Autodesk Inventor part; units mm, degrees
ref_plane "YZ Plane" through (0, 0, 0) normal (1, 0, 0) x (0, 1, 0)
ref_plane "XZ Plane" through (0, 0, 0) normal (0, 1, 0) x (-1, 0, 0)
ref_plane "XY Plane" through (0, 0, 0) normal (0, 0, 1) x (1, 0, 0)
sketch "Sketch1" plane through (0, 0, 0) normal (0, 0, 1) x (1, 0, 0)
  line L0 (0.0426, 8.3509) -> (2.1366, 8.3509) construction
  line L1 (-5.93, 6.5274) -> (-3.3043, 9.5646)
  line L2 (-3.3043, 9.5646) -> (-1.75, 9.5646)
  line L3 (-1.75, 9.5646) -> (-1.75, 6.9793)
  line L4 (-1.75, 6.9793) -> (0, 8.1293)
  line L5 (0, 8.1293) -> (0, 0)
  line L6 (0, 0) -> (-1.75, 1.15)
  line L7 (-1.75, 1.15) -> (-1.75, -1.4354)
  line L8 (-1.75, -1.4354) -> (-3.3043, -1.4354)
  line L9 (-3.3043, -1.4354) -> (-5.93, 1.6019)
  line L10 (-5.93, 1.6019) -> (-5.93, 6.5274)
  dimension "d16" = 0
  dimension "d17" = 0
extrude "Extrusion1" add sketch "Sketch1" along normal blind 164.9
sketch "Sketch2" plane through (0, 0, 0) normal (1, 0, 0) x (0, 0, -1)
  line L0 (0, 8.1293) -> (-164.9, 8.1293)
  line L1 (0, 0) -> (0, 8.1293)
  line L2 (-164.9, 8.1293) -> (0, 8.1293)
  line L3 (0, 8.1293) -> (0, 0)
  line L4 (0, 0) -> (-164.9, 0)
  line L5 (-164.9, 0) -> (-164.9, 8.1293)
extrude "Extrusion2" add sketch "Sketch2" along normal blind 1
sketch "Sketch3" plane through (1, 0, 0) normal (1, 0, 0) x (0, 0, -1)
  line L0 (-164.9, 8.1293) -> (-164.9, 0)
  line L1 (0, 2.065) -> (-164.9, 2.065)
  line L2 (-164.9, 2.065) -> (-164.9, 6.065)
  line L3 (-164.9, 6.065) -> (0, 6.065)
  line L4 (0, 6.065) -> (0, 2.065)
  line L5 (0, 2.065) -> (-164.9, 6.065) construction
  line L6 (-164.9, 2.065) -> (0, 6.065) construction
  line L7 (0, 0) -> (0, 8.1293)
  point P0 (-82.45, 4.065)
  dimension "d22" = 4
  dimension "d28" = 0
extrude "Extrusion3" add sketch "Sketch3" along normal blind 10.5
sketch "Sketch4" plane through (1, 2.065, 0) normal (0, -1, 0) x (1, 0, 0)
  point P0 (-1, 0)
sketch "Sketch5" plane through (1, 2.065, 0) normal (0, -1, 0) x (1, 0, 0)
  line L0 (0, 164.9) -> (10.5, 164.9)
  line L1 (9.5, -0.1) -> (1, -0.1)
  line L2 (1, -0.1) -> (1, 164.9)
  line L3 (1, 164.9) -> (9.5, 164.9)
  line L4 (9.5, 164.9) -> (9.5, -0.1)
  line L5 (9.5, -0.1) -> (1, 164.9) construction
  line L6 (1, -0.1) -> (9.5, 164.9) construction
  point P0 (-1, 0)
  point P1 (5.25, 82.4)
  dimension "d25" = 8.5
extrude "Extrusion4" cut sketch "Sketch5" against normal blind 0.9
fillet "Fillet1" radius 2 1 edges at (11.5, 6.065, 82.45)
fillet "Fillet2" radius 0.2 1 edges at (10.5, 2.965, 82.45)
fillet "Fillet3" radius 0.2 1 edges at (2, 2.965, 82.45)
fillet "Fillet4" radius 0.2 3 edges at (11.5, 2.065, 82.45) (10.5, 2.065, 82.45) (2, 2.065, 82.45)
properties part number "LED Strip Top Mount"
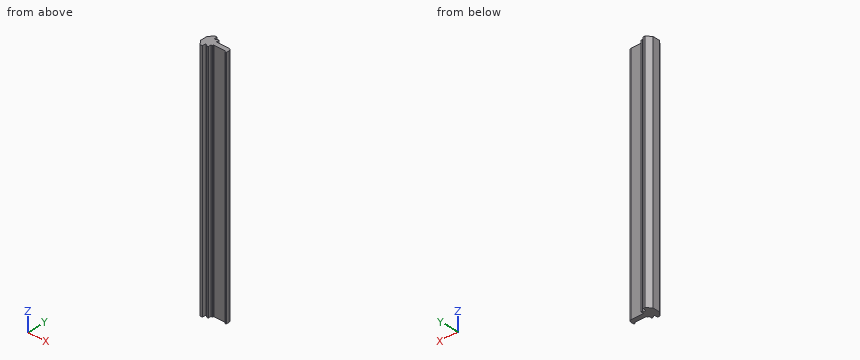
CAD build for the part. Positions are in the model's coordinates, mm. Round coordinates to 2 decimals unless told otherwise and drop trailing zeros. Loops run counter-clockwise (first coordinate to the right, second up) from the corner with the lowest first, then second, coordinate; pieces in that order, holes last.
(1) Drop flat-ended pins along their axis: pin 1 (2 mm diameter, centred on y = 8.5, z = 70.5, fed in from +X); pin 2 (3 mm diameter, centred on x = 0, z = 38.5, fed in from +Y); pin 3 (7 mm diameter, centred on x = 7, z = 47.5, fed in from +Y) (3 decimals). Give the stop position or say it passes through.
(2) Cut at A-A (z = 52). Give the cut face in (x, y) (3 decimals).
(3) Wall check: line 1 along X through (y, z) = (7.5, 21); line 2 along X through (y, z) = (0.5, 119); line 3 along X through (y, z) = (2, 68). Give the ranges that are in metal, low to high.
(4) Cut at B-B (x = 7.75). Give the cut face in (y, z) (3 decimals).
Findings below:
1. pin 1: stops at x = 1
1. pin 2: stops at y = 8.13
1. pin 3: stops at y = 6.065
2. outline: (-5.93, 1.602) - (-3.304, -1.435) - (-1.75, -1.435) - (-1.75, 1.15) - (0, 0) - (1, 0) - (1, 2.065) - (1.8, 2.065) arc R0.2 ccw to (2, 2.265) - (2, 2.765) arc R0.2 cw to (2.2, 2.965) - (10.3, 2.965) arc R0.2 cw to (10.5, 2.765) - (10.5, 2.265) arc R0.2 ccw to (10.7, 2.065) - (11.3, 2.065) arc R0.2 ccw to (11.5, 2.265) - (11.5, 4.065) arc R2 ccw to (9.5, 6.065) - (1, 6.065) - (1, 8.129) - (0, 8.129) - (-1.75, 6.979) - (-1.75, 9.565) - (-3.304, 9.565) - (-5.93, 6.527) - close
3. line 1: x = -5.09 to -1.75, -0.96 to 1
3. line 2: x = -4.98 to -1.75, -0.76 to 1
3. line 3: x = -5.93 to 1
4. outline: (2.965, 0) - (6.065, 0) - (6.065, 164.9) - (2.965, 164.9) - close
